The listing builds one solid part. Answer for the finished solid, in the listing's coordinates (mm). Face numbers are marked on the shaded views. A direction names the side the tool comes from. Give positions to 0.01 mm unless a question says otherwise; leave off trailing zeros. Write each loop counter-clockwise with the first axis right and the second up, starting at its lowest first coordinate (ties: lowest second). Pieces come first, ordered by that corner, then holes.
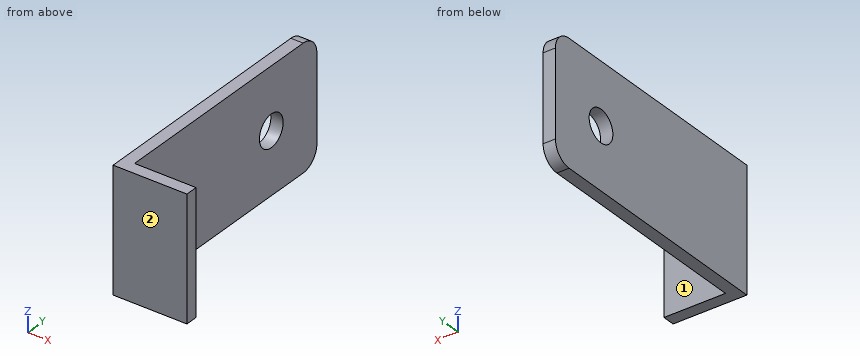
```python
from build123d import *

# Parameters (mm, degrees)
EXTRUDE_1_DEPTH     = 20
SKETCH_2_R          = 2.6
CUT_EXTRUDE_1_DEPTH = 10
FILLET_1_R          = 3


with BuildPart() as part:
    # 草图1 → 拉伸-薄壁1 (new body)
    with BuildSketch(Plane.XY):
        Polygon((0, 40), (0, 0), (10, 0), (10, -2), (-2, -2), (-2, 40), align=None)
    extrude(amount=EXTRUDE_1_DEPTH)

    # 草图2 → 切除-拉伸1 (cut)
    with BuildSketch(Plane(origin=(0, 0, 0), x_dir=(0, 0, -1), z_dir=(1, 0, 0))):
        with Locations((-10, 30)):
            Circle(SKETCH_2_R)
    extrude(amount=-CUT_EXTRUDE_1_DEPTH, mode=Mode.SUBTRACT)

    # 圆角1
    fillet_1_edges = [part.edges().sort_by_distance(p)[0] for p in [
        (-1, 40, 20),
        (-1, 40, 0),
    ]]
    fillet(fillet_1_edges, radius=FILLET_1_R)


solid = part.part
```
Item 1: Each of these flat-tipped pins is pushed along its axis until it touches: P1, Ø6, axis at x = 8, z = 5.5, coming from the +Y side; P2, Ø6, axis at y = 30, z = 10, coming from the +X side. Where does it stop, or does it pass through?
Conclusion:
P1: stops at y = 0
P2: stops at x = 0
Item 2: A cutting plane is placed at A-A, the plane y = 30. Give the vertices of the cut face in (x, z), plus the area to 3 significant figures.
Conclusion:
outline: (-2, 0) - (0, 0) - (0, 7.4) - (-2, 7.4) - close; (-2, 12.6) - (0, 12.6) - (0, 20) - (-2, 20) - close
area: 29.6 mm2
Item 3: A cutting plane is placed at B-B, the plane z = 10. Give the vertices of the cut face in (x, y).
Conclusion:
outline: (-2, -2) - (10, -2) - (10, 0) - (0, 0) - (0, 27.4) - (-2, 27.4) - close; (-2, 32.6) - (0, 32.6) - (0, 40) - (-2, 40) - close
Item 4: A cutting plane is placed at C-C, the plane x = -0.5. Give the vertices of the cut face in (y, z), plus the area to 3 significant figures.
Conclusion:
outline: (-2, 0) - (37, 0) arc R3 ccw to (40, 3) - (40, 17) arc R3 ccw to (37, 20) - (-2, 20) - close; hole circle Ø5.2 at (30, 10)
area: 815 mm2
Item 5: Which of the six approach directions +Z, -Z, +X, -X, +Y, -Y give full straight-line access (tool end or side, diameter ignored) to the marked faces 1 and 2?
Conclusion:
face 1: +Z, -Z, +X, +Y
face 2: +Z, -Z, +X, -X, -Y
Item 6: Consider probe 1 along Y at (x, z) = (-0.75, 10); probe 2 along X at (y, z) = (26.5, 17.75). Determine where each line is inside the solid, lowest interval first.
Conclusion:
probe 1: y = -2 to 27.4, 32.6 to 40
probe 2: x = -2 to 0
Item 7: A cutting plane is placed at D-D, the plane z = 3.75. Give the vertices of the cut face in (x, y), plus the area to 3 significant figures.
Conclusion:
outline: (-2, -2) - (10, -2) - (10, 0) - (0, 0) - (0, 40) - (-2, 40) - close
area: 104 mm2
